Check sheet for the modelled part. Datum: model origin and axes. Units: mm. Face numbers are marked on the shaded views. A direction names the side the tool comes from. Give positions to 0.01 mm unless a question says otherwise; leave off trailing zeros. Loops run counter-clockwise (first coordinate to the right, second up) from the corner with the lowest first, then second, coordinate; pieces in that order, holes last. Notation, with made-up numbers: (-18.5, 2.25) - (8.5, 2.25) arc R12 cw to (8.5, 7.25) - close; hole circle Ø10 at (79, 48.5). An arc over 180 degrees is marked (long way). Use CSV: the item, a comma, the result in double quotes.
from build123d import *

# Parameters (mm, degrees)
F0_R     = 10.95
F1_DEPTH = 10


with BuildPart() as f1:
    # F0 (on Front) → F1 (new body)
    with BuildSketch(Plane.XZ):
        with BuildLine():
            Line((-6.227786, 41.574522), (-15.947611, 14.116478))
            Line((-15.947611, 14.116478), (-41.427071, 5.794421))
            ThreePointArc((-41.427071, 5.794421), (-45.805064, -0.163891), (-41.574522, -6.227786))
            Line((-41.574522, -6.227786), (-14.116478, -15.947611))
            Line((-14.116478, -15.947611), (-5.794421, -41.427071))
            ThreePointArc((-5.794421, -41.427071), (0.163891, -45.805064), (6.227786, -41.574522))
            Line((6.227786, -41.574522), (15.947611, -14.116478))
            Line((15.947611, -14.116478), (41.427071, -5.794421))
            ThreePointArc((41.427071, -5.794421), (45.805064, 0.163891), (41.574522, 6.227786))
            Line((41.574522, 6.227786), (14.116478, 15.947611))
            Line((14.116478, 15.947611), (5.794421, 41.427071))
            ThreePointArc((5.794421, 41.427071), (-0.163891, 45.805064), (-6.227786, 41.574522))
        make_face()
        Polygon((-5.45, -23.189698), (0, -20.043139), (5.45, -23.189698), (5.45, -29.482816), (0, -32.629375), (-5.45, -29.482816), align=None, mode=Mode.SUBTRACT)
        Polygon((-23.189698, 5.45), (-20.043139, 0), (-23.189698, -5.45), (-29.482816, -5.45), (-32.629375, 0), (-29.482816, 5.45), align=None, mode=Mode.SUBTRACT)
        Circle(F0_R, mode=Mode.SUBTRACT)
        Polygon((0, 32.629375), (5.45, 29.482816), (5.45, 23.189698), (0, 20.043139), (-5.45, 23.189698), (-5.45, 29.482816), align=None, mode=Mode.SUBTRACT)
        Polygon((23.189698, -5.45), (20.043139, 0), (23.189698, 5.45), (29.482816, 5.45), (32.629375, 0), (29.482816, -5.45), align=None, mode=Mode.SUBTRACT)
    extrude(amount=F1_DEPTH)


solid = f1.part
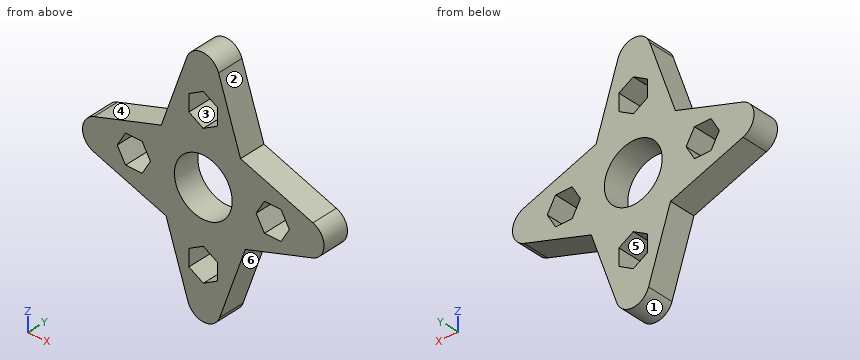
1. Sectioned sample at B-B, the plane z = 25. Record the boundary of the cut face in (x, y).
Completed:
outline,"(-12.09, -10) - (-5.45, -10) - (-5.45, 0) - (-12.09, 0) - close; (5.45, -10) - (11.16, -10) - (11.16, 0) - (5.45, 0) - close"
2. Scan lines: line 1 along Z through (x, y) = (0, -6.5); line 2 along Z through (x, y) = (-5, -9.5); line 3 along X through (y, z) = (-7.5, -4). Record each from-to range of solid material in increasing order.
Completed:
line 1,"z = -45.8 to -32.63, -20.04 to -10.95, 10.95 to 20.04, 32.63 to 45.8"
line 2,"z = -43.04 to -29.74, -22.93 to -9.74, 9.74 to 22.93, 29.74 to 43.66"
line 3,"x = -44.57 to -30.32, -22.35 to -10.19, 10.19 to 22.35, 30.32 to 44.18"
3. Release check for a two-part mould opening along X. For the marked faces 1, 2, 3 and 4 record: released by +X, released by -X, zero draft, split by the parting line, or undercut.
Completed:
face 1,"split by the parting line"
face 2,"released by +X"
face 3,"undercut"
face 4,"released by -X"
4. Sectioned sample at D-D, the plane z = -35. Record the boundary of the cut face in (x, y), and give its area (3 significant figures).
Completed:
outline,"(-7.89, -10) - (8.56, -10) - (8.56, 0) - (-7.89, 0) - close"
area,"164 mm²"
5. Set-up check for the marked faces 5 and 6: record each of +Z, -Z, +X, -X, +Y, -Y from which the full face is reachable in a straight line by a thin tool's end or side.
Completed:
face 5,"+Y, -Y"
face 6,"-Z, +X, +Y, -Y"
6. Go/stop test with flat-tipped pins: pin 1 Ø1.9 at (x, y) = (-27, -4) entering from +Z; pin 2 Ø1.9 at (x, y) = (27.5, -4.5) entering from -Z; pin 3 Ø2 at (y, z) = (-2, -22.5) entering from +X; pin 4 Ø3 at (x, z) = (-0.5, -29) entering from -Y. Record where each tip stops, or that it passes through.
Completed:
pin 1,"stops at z = 10.82"
pin 2,"stops at z = -10.65"
pin 3,"stops at x = 13.33"
pin 4,"passes through"
7. Sectioned sample at C-C, the plane y = -4. State how many separate pieces and enclosed holes the cut face has, and give its area (3 significant figures).
Completed:
separate pieces,"1"
enclosed holes,"5"
area,"2,500 mm²"
8. Sectioned sample at A-A, the plane x = -4. Record the boundary of the cut face in (y, z).
Completed:
outline,"(-10, -44.18) - (0, -44.18) - (0, -30.32) - (-10, -30.32) - close; (-10, -22.35) - (0, -22.35) - (0, -10.19) - (-10, -10.19) - close; (-10, 10.19) - (0, 10.19) - (0, 22.35) - (-10, 22.35) - close; (-10, 30.32) - (0, 30.32) - (0, 44.57) - (-10, 44.57) - close"
